The figure shows three views and two pictorial views of one solid part (mm, origin at its lowest corner). Answer the questions. A direction names the side the tool comes from. Round coordinates to 2 decimals unless told otherwise and drop trailing zeros. Order: outer loops, then holes, each group sorted by start corner. A loop starts at its lowest first (then second) coordinate and runs counter-clockwise, first axis right, second up. Notation, with made-up numbers: M 51.25,8.5 L 85.25,8.5 A17 ccw 85.25,35.5 Z; hole C 42,75 d10. An arc over 180 degrees is marked long. Return JSON: item names as keys, results as strings.
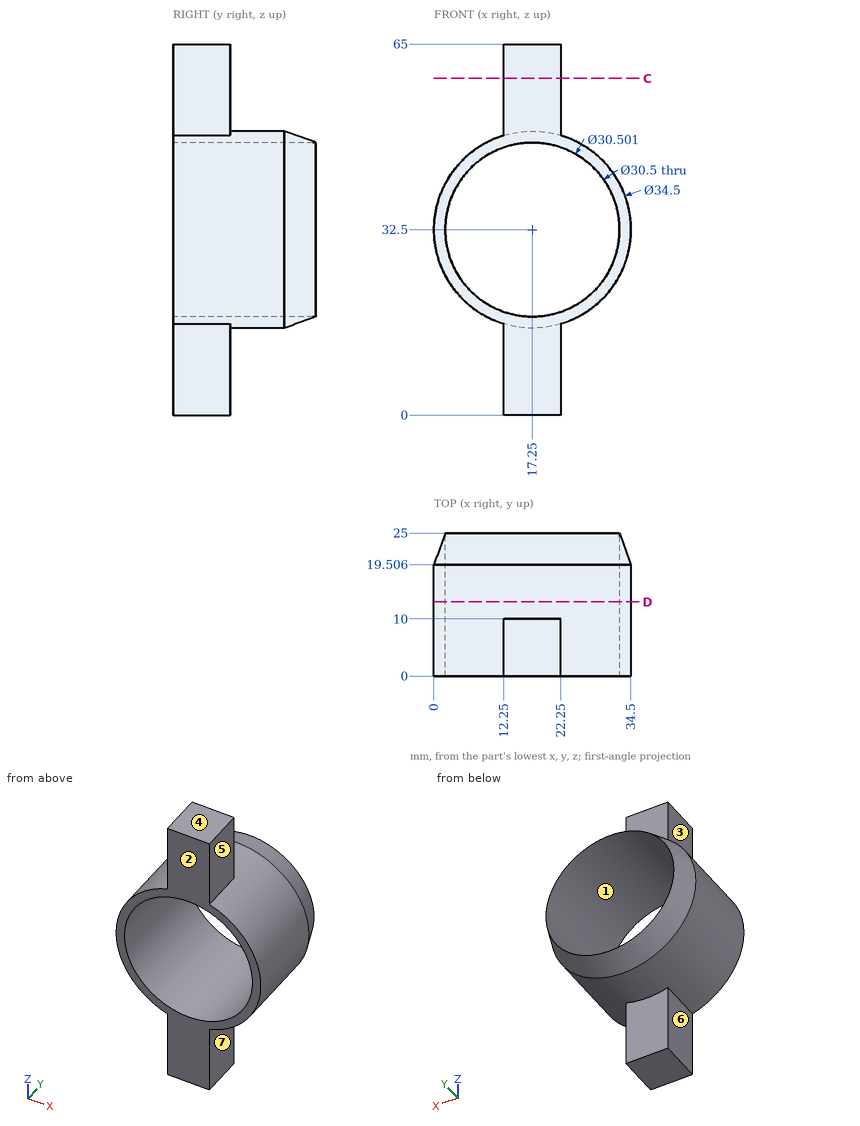
Item 1: The mould has two halves that part along X. Classify the marked faces 1, 2 and 3: pulls with the +X half, pulls with the -X half, needs draft (parallel to the pull), parting line crosses it, or undercut.
Output:
{"face 1": "undercut", "face 2": "needs draft", "face 3": "pulls with the -X half"}
Item 2: Consider line 1 along Z through (x, y) = (17.25, 19.5); line 2 along Z through (x, y) = (17.25, 5.25); line 3 along X through (y, z) = (8.25, 54). Determine where each line is inside the solid, lowest interval first. Write a range as [from, to].
Output:
{"line 1": "z = [15.25, 17.25], [47.75, 49.75]", "line 2": "z = [0, 17.25], [47.75, 65]", "line 3": "x = [12.25, 22.25]"}
Item 3: Each of these flat-tipped pins is pushed along its axis until it touches: pin 1 (3 mm diameter, centred on y = 7.5, z = 4, fed in from +X); pin 2 (10 mm diameter, centred on y = 9.5, z = 40.5, fed in from -X); pin 3 (3 mm diameter, centred on x = 15.5, z = 54, fed in from +Y). Where does it stop, or does it pass through?
Output:
{"pin 1": "stops at x = 22.25", "pin 2": "stops at x = 0.26", "pin 3": "stops at y = 10"}
Item 4: Find section D-D (y = 13). Determine the outline of the cut face in (x, z), plus the area to 3 significant figures.
Output:
{"outline": "C 17.25,32.5 d34.5; hole C 17.25,32.5 d30.5", "area": "204 mm^2"}
Item 5: Find section C-C (z = 59). Determine the outline of the cut face in (x, y), plus the area to 3 significant figures.
Output:
{"outline": "M 12.25,0 L 22.25,0 L 22.25,10 L 12.25,10 Z", "area": "100 mm^2"}
Item 6: Which of the six approach directions +Z, -Z, +X, -X, +Y, -Y give full straight-line access (tool end or side, diameter ignored) to the marked faces 4, 5, 6 and 7?
Output:
{"face 4": "+Z, +X, -X, +Y, -Y", "face 5": "+Z, +X, +Y, -Y", "face 6": "-Z, -X, +Y, -Y", "face 7": "-Z, +X, +Y, -Y"}
